Source: CAD feature listing. Evaluate the final solid. Frame: model axes, mm. Face numbers are marked on the shaded views. A direction names the side the tool comes from. Round coordinates to 2 decimals unless told otherwise and drop trailing zeros. Loops run counter-clockwise (first coordinate to the right, second up) from the corner with the lowest first, then second, coordinate; pieces in that order, holes last.
(1) Material intervals for probe 1 along Y at (x, z) = (3, 3.25); probe 2 along Y at (x, z) = (2, 1.5); probe 3 along X at (y, z) = (-1.5, 8), sorted ascending.
(2) Section A-A, the plane x = 0. Return the cut outline in (y, z), plus the area to 3 significant figures.
(3) Set-up query: the marked faces 1 and 2. Return all of +Z, -Z, +X, -X, +Y, -Y with unobstructed straight access to the full face (end or side cutting, diameter ignored); none if empty.
(4) Section C-C, the plane z = 7.75. Return the cut outline in (x, y).
(5) First-contact query: pin 1 Ø3 at (y, z) = (0.5, 9.5) entering from +X; pin 2 Ø1.5 at (x, z) = (-1.5, 8) entering from +Y. Flat tips, straight axial feed; report the tip coordinate or a pass-through.
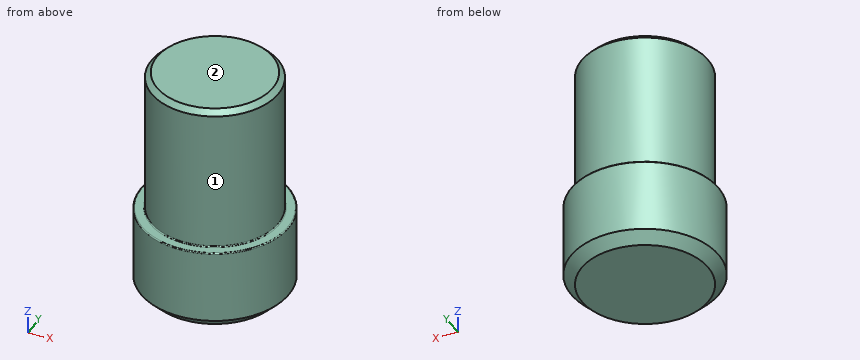
```python
from build123d import *

# Parameters (mm, degrees)
SCHIZZO1_R                   = 3.5
ESTRUSIONE_ESTRUSIONE1_DEPTH = 4
SCHIZZO2_R                   = 3
ESTRUSIONE_ESTRUSIONE2_DEPTH = 7
SMUSSO1_SIZE                 = 0.25
SMUSSO2_SIZE                 = 0.5
RACCORDO1_R                  = 0.05


with BuildPart() as part:
    # Schizzo1 → Estrusione-Estrusione1 (new body)
    with BuildSketch(Plane.XY):
        Circle(SCHIZZO1_R)
    extrude(amount=ESTRUSIONE_ESTRUSIONE1_DEPTH)

    # Schizzo2 → Estrusione-Estrusione2 (add)
    with BuildSketch(Plane.XY.offset(4)):
        Circle(SCHIZZO2_R)
    extrude(amount=ESTRUSIONE_ESTRUSIONE2_DEPTH)

    # Smusso1
    smusso1_edges = [part.edges().sort_by_distance(p)[0] for p in [
        (-3, 0, 11),
    ]]
    chamfer(smusso1_edges, length=SMUSSO1_SIZE)

    # Smusso2
    smusso2_edges = [part.edges().sort_by_distance(p)[0] for p in [
        (-3.5, 0, 0),
    ]]
    chamfer(smusso2_edges, length=SMUSSO2_SIZE)

    # Raccordo1
    raccordo1_edges = [part.edges().sort_by_distance(p)[0] for p in [
        (-3.5, 0, 4),
        (-3, 0, 4),
    ]]
    fillet(raccordo1_edges, radius=RACCORDO1_R)


solid = part.part
```
Output values:
1. probe 1: y = -1.8 to 1.8
1. probe 2: y = -2.87 to 2.87
1. probe 3: x = -2.6 to 2.6
2. outline: (-3.5, 0.5) - (-3, 0) - (3, 0) - (3.5, 0.5) - (3.5, 3.95) arc R0.05 ccw to (3.45, 4) - (3.05, 4) arc R0.05 cw to (3, 4.05) - (3, 10.75) - (2.75, 11) - (-2.75, 11) - (-3, 10.75) - (-3, 4.05) arc R0.05 cw to (-3.05, 4) - (-3.45, 4) arc R0.05 ccw to (-3.5, 3.95) - close
2. area: 69.7 mm2
3. face 1: +Z
3. face 2: +Z, +X, -X, +Y, -Y
4. outline: circle Ø6 at (0, 0)
5. pin 1: stops at x = 3
5. pin 2: stops at y = 2.9
